```python
from build123d import *

# Parameters (mm, degrees)
PAD_DEPTH       = 14
POCKET_DEPTH    = 13.5
SKETCH002_R     = 1.5
POCKET001_DEPTH = 14.001


with BuildPart() as part:
    # Sketch → Pad (new body)
    with BuildSketch(Plane.XZ):
        with BuildLine():
            Line((-3.5, 5), (3.5, 5))
            ThreePointArc((6, 1), (5.323594, 3.358497), (3.5, 5))
            Line((6, 1), (6, -1))
            ThreePointArc((3.5, -5), (5.323594, -3.358497), (6, -1))
            Line((-3.5, -5), (3.5, -5))
            ThreePointArc((-6, -1), (-5.323594, -3.358496), (-3.5, -5))
            Line((-6, 1), (-6, -1))
            ThreePointArc((-3.5, 5), (-5.323594, 3.358496), (-6, 1))
        make_face()
    extrude(amount=PAD_DEPTH)

    # Sketch001 → Pocket (cut)
    with BuildSketch(Plane.XZ):
        with BuildLine():
            Line((-3, 4.5), (3, 4.5))
            ThreePointArc((5.5, 1), (4.810812, 3.15058), (3, 4.5))
            Line((5.5, 1), (5.5, -1))
            ThreePointArc((3, -4.5), (4.810812, -3.15058), (5.5, -1))
            Line((-3, -4.5), (3, -4.5))
            ThreePointArc((-5.5, -1), (-4.810812, -3.15058), (-3, -4.5))
            Line((-5.5, -1), (-5.5, 1))
            ThreePointArc((-3, 4.5), (-4.810812, 3.15058), (-5.5, 1))
        make_face()
    extrude(amount=POCKET_DEPTH, mode=Mode.SUBTRACT)

    # Sketch002 → Pocket001 (cut, through all)
    with BuildSketch(Plane.XZ):
        Circle(SKETCH002_R)
    extrude(amount=POCKET001_DEPTH, mode=Mode.SUBTRACT)


solid = part.part
```
For this review, take the finished solid that the model builds, in its own axes (mm). A direction names the side the tool comes from. Coordinates: 2 decimals unless noted, no trailing zeros. Loops run counter-clockwise (first coordinate to the right, second up) from the corner with the lowest first, then second, coordinate; pieces in that order, holes last. Notation, with made-up numbers: (10.25, -21.5) - (30.25, -21.5) arc R17 cw to (30.25, 3.5) - close; hole circle Ø6 at (2, 8.5). An arc over 180 degrees is marked (long way). Use one line per item in the form item = value. Start each with the question number.
1) Take a section at A-A (x = 0). State the section outline as (y, z) points, plus the area to 3 significant figures.
2) To check wall thickness, follow probe 1 along Z at (x, y) = (0, -13.65); probe 2 along X at (y, z) = (-5.5, 0); probe 3 along Z at (x, y) = (1.5, -8.5). State the ranges of each line that lie inside material, in increasing order. Write a range as from..to.
3) Take a section at B-B (z = 0). State the section outline as (x, y) points.
4) For faces 5 (the face through (-5.34, -6.9, -3.33)), 6 (the face through (4.83, -6.66, 3.12)), list the 3-axis set-ups (+Z, -Z, +X, -X, +Y, -Y) from which the entire face can be reached by the end or side of a thin tool; tool diameter is ignored.
5) Take a section at D-D (x = 2). State the section outline as (y, z) points.
6) Take a section at C-C (y = -8). State the section outline as (x, z) points, plus the area to 3 significant figures.
7) Draft analysis for pull direction Z (two halves, no side actions). For faces 1 (the face through (-5.305, -6.902, 3.388)), 2 (the face through (4.79, -6.66, -3.18)), 3 (the face through (-4.79, -6.66, 3.18)), 4 (the face through (0, 0, 4.8)), state which applies: released by +Z, released by -Z, zero draft, split by the parting line, or undercut.
8) For pin 1 (2.5 mm diameter, centred on x = 2.5, z = 0, fed in from +Y); pin 2 (5 mm diameter, centred on y = -3.5, z = -4, fed in from +X), all flat-tipped, find the tip position at first contact; note any pin that passes through.
From the geometry:
q1.outline = (-14, -5) - (0, -5) - (0, -4.5) - (-13.5, -4.5) - (-13.5, -1.5) - (-14, -1.5) - close; (-14, 1.5) - (-13.5, 1.5) - (-13.5, 4.5) - (0, 4.5) - (0, 5) - (-14, 5) - close
q1.area = 17.0 mm2
q2.probe_1 = -5..-1.5, 1.5..5
q2.probe_2 = -6..-5.5, 5.5..6
q2.probe_3 = -5..-4.5, 4.5..5
q3.outline = (-6, -14) - (-1.5, -14) - (-1.5, -13.5) - (-5.5, -13.5) - (-5.5, 0) - (-6, 0) - close; (1.5, -14) - (6, -14) - (6, 0) - (5.5, 0) - (5.5, -13.5) - (1.5, -13.5) - close
q4.face_5 = -Z, -X, +Y, -Y
q4.face_6 = +Y
q5.outline = (-14, -5) - (0, -5) - (0, -4.5) - (-13.5, -4.5) - (-13.5, 4.5) - (0, 4.5) - (0, 5) - (-14, 5) - close
q6.outline = (-6, -1) arc R4.45 ccw to (-3.5, -5) - (3.5, -5) arc R4.45 ccw to (6, -1) - (6, 1) arc R4.45 ccw to (3.5, 5) - (-3.5, 5) arc R4.45 ccw to (-6, 1) - close; hole (-5.5, -1) arc R3.7 ccw to (-3, -4.5) - (3, -4.5) arc R3.7 ccw to (5.5, -1) - (5.5, 1) arc R3.7 ccw to (3, 4.5) - (-3, 4.5) arc R3.7 ccw to (-5.5, 1) - close
q6.area = 19.1 mm2
q7.face_1 = released by +Z
q7.face_2 = undercut
q7.face_3 = undercut
q7.face_4 = zero draft
q8.pin_1 = -13.5
q8.pin_2 = 5.97
